Source: CAD feature listing. Evaluate the final solid. Frame: model axes, mm. Round coordinates to 2 decimals unless told otherwise and drop trailing zeros. Order: outer loops, then holes, each group sorted by start corner. A loop starts at its lowest first (then second) coordinate and runs counter-clockwise, first axis right, second up. Notation, with made-up numbers: (58.5, 24) - (108.5, 24) arc R21 cw to (108.5, 37) - close; hole circle Ø4 at (15.25, 14.5). An arc over 180 degrees is marked (long way). Return JSON: item names as keys, results as strings. Group by question number.
1) Ray query, line 1 (Y direction, x = -28.5, z = 1.9); line 2 (X direction, y = 66.5, z = 3.1); line 3 (Y direction, x = 29.36, z = 3.4). Return the intervals inside material, ascending. Write a range as from..to.
2) Contact query for flat-ended pins moving along their axis: P1, Ø1, axis at y = 46.5, z = 1.5, coming from the +X side; P2, Ø4.5, axis at x = -28.16, y = 46.39, coming from the -Z side. Output: stop coordinate, or through.
3) Section D-D, the plane y = 46.39. Return loops of the section in (x, z).
4) Section B-B, the plane y = -68.49. Return loops of the section in (x, z), plus the area to 3 significant figures.
5) Mould query, pull axis Y, two halves, no side actions, for faces 1 (the cylindrical face through (-10.73, 81.72, 2.46)), 2 (the cylindrical face through (29.03, -66.01, 2.54)), 3 (the flat face through (-1, 1, 5)). Classes: pulls with the +Y half, pulls with the -Y half, needs draft (parallel to the pull), parting line crosses it, or undercut.
6) Section A-A, the plane z = 2.5. Give the number of separate pieces and of enclosed holes in the cut face, plus the area to 3 significant figures.
7) Section C-C, the plane x = -28.16. Return loops of the section in (y, z).
```python
from build123d import *

# Parameters (mm, degrees)
CROQUIS1_R              = 82.42
SALIENTE_EXTRUIR1_DEPTH = 5
CROQUIS3_R              = 2.5
CORTAR_EXTRUIR1_DEPTH   = 5


with BuildPart() as part:
    # Croquis1 → Saliente-Extruir1 (new body)
    with BuildSketch(Plane.XY):
        Circle(CROQUIS1_R)
    extrude(amount=SALIENTE_EXTRUIR1_DEPTH)

    # Croquis3 → Cortar-Extruir1 (cut, symmetric)
    with BuildSketch(Plane.XY.offset(5)):
        with Locations((29.36, 46.39)):
            Circle(CROQUIS3_R)
        with Locations((-28.16, 68.49)):
            Circle(CROQUIS3_R)
        with Locations((29.36, -46.39)):
            Circle(CROQUIS3_R)
        with Locations((-28.16, -46.39)):
            Circle(CROQUIS3_R)
        with Locations((29.36, -68.49)):
            Circle(CROQUIS3_R)
        with Locations(Location((29.36, 68.49, 0), (0, 0, 180))):
            Circle(CROQUIS3_R)
        with Locations(Location((-28.16, 46.39, 0), (0, 0, 180))):
            Circle(CROQUIS3_R)
        with Locations((-28.16, -68.49)):
            Circle(CROQUIS3_R)
    extrude(amount=CORTAR_EXTRUIR1_DEPTH, both=True, mode=Mode.SUBTRACT)


solid = part.part
```
Geometry check:
{
 "1": {"line 1": "-77.34..-70.97, -66.01..-48.87, -43.91..43.91, 48.87..66.01, 70.97..77.34", "line 2": "-48.69..-29.67, -26.65..27.85, 30.87..48.69", "line 3": "-77.01..-70.99, -65.99..-48.89, -43.89..43.89, 48.89..65.99, 70.99..77.01"},
 "2": {"P1": "x = 68.39", "P2": "through"},
 "3": {"outline": "(-68.13, 0) - (-30.66, 0) - (-30.66, 5) - (-68.13, 5) - close; (-25.66, 0) - (26.86, 0) - (26.86, 5) - (-25.66, 5) - close; (31.86, 0) - (68.13, 0) - (68.13, 5) - (31.86, 5) - close"},
 "4": {"outline": "(-45.85, 0) - (-30.66, 0) - (-30.66, 5) - (-45.85, 5) - close; (-25.66, 0) - (26.86, 0) - (26.86, 5) - (-25.66, 5) - close; (31.86, 0) - (45.85, 0) - (45.85, 5) - (31.86, 5) - close", "area": "408 mm2"},
 "5": {"face 1": "parting line crosses it", "face 2": "undercut", "face 3": "needs draft"},
 "6": {"separate pieces": "1", "enclosed holes": "8", "area": "21,200 mm2"},
 "7": {"outline": "(-77.46, 0) - (-70.99, 0) - (-70.99, 5) - (-77.46, 5) - close; (-65.99, 0) - (-48.89, 0) - (-48.89, 5) - (-65.99, 5) - close; (-43.89, 0) - (43.89, 0) - (43.89, 5) - (-43.89, 5) - close; (48.89, 0) - (65.99, 0) - (65.99, 5) - (48.89, 5) - close; (70.99, 0) - (77.46, 0) - (77.46, 5) - (70.99, 5) - close"}
}
